The listing builds one solid part. Answer for the finished solid, in the listing's coordinates (mm). A direction names the side the tool comes from. Coordinates: 2 decimals unless noted, no trailing zeros. Loops run counter-clockwise (first coordinate to the right, second up) from the corner with the lowest first, then second, coordinate; pieces in that order, holes last. Notation, with made-up numbers: (-9.5, 0.5) - (36.5, 0.5) arc R26 ccw to (36.5, 28.5) - close; hole circle Ø11 at (-33.5, 42). An arc over 180 degrees is marked (long way). Return JSON: item names as keys, results as strings. Group by question number.
1. Section B-B (z = 402) is taken. Write down the section's boundary in (x, y), and give its area (3 significant figures).
2. Which of the six approach directions +Z, -Z, +X, -X, +Y, -Y give full straight-line access (tool end or side, diameter ignored) to faces 4 (the face through (31.75, 16, 363)), 5 (the face through (6.35, 16, 363))?
3. Find the intervals of material crossed by line 1 along X through (y, z) = (20.5, 138.5); line 2 along Z through (x, y) = (15.5, 26.5), in increasing order.
4. The mould has two halves that part along Y. Classify faces 1 (the face through (0, 16, 363)), 2 (the face through (16, 25.4, 363)), 3 (the face through (16, 31.75, 363)): pulls with the +Y half, pulls with the -Y half, needs draft (parallel to the pull), parting line crosses it, or undercut.
5. Each of these flat-tipped pins is pushed along its axis until it touches: P1, Ø7.5, axis at x = 15.875, z = 25.4, coming from the -Y side; P2, Ø8, axis at x = 8.5, y = 8.5, coming from the -Z side. Where does it stop, or does it pass through?
```python
from build123d import *

# Parameters (mm, degrees)
F0_W     = 31.75
F0_H     = 31.75
F0_W_2   = 19.05
F0_H_2   = 19.05
F1_DEPTH = 736.6
F2_R     = 4.7625
F3_DEPTH = 31.751
F5_DEPTH = 31.751


with BuildPart() as f1:
    # F0 (on Top) → F1 (new body)
    with BuildSketch(Plane.XY):
        with Locations((15.875, 15.875)):
            Rectangle(F0_W, F0_H)
        with Locations((15.875, 15.875)):
            Rectangle(F0_W_2, F0_H_2, mode=Mode.SUBTRACT)
    extrude(amount=F1_DEPTH)

    # F2 (on face) → F3 (cut, through all)
    with BuildSketch(Plane.XZ):
        with Locations((15.875, 25.4)):
            Circle(F2_R)
    extrude(amount=-F3_DEPTH, mode=Mode.SUBTRACT)

    # F4 (on face) → F5 (cut, through all)
    with BuildSketch(Plane.XZ):
        with BuildLine():
            ThreePointArc((27.532244, 727.619744), (27.16972, 729.442274), (26.13734, 730.98734))
            ThreePointArc((26.13734, 730.98734), (18.369768, 725.797214), (27.532244, 727.619744))
        make_face()
    extrude(amount=-F5_DEPTH, mode=Mode.SUBTRACT)


solid = f1.part
```
The answers:
{
 "1": {"outline": "(0, 0) - (31.75, 0) - (31.75, 31.75) - (0, 31.75) - close; hole (6.35, 6.35) - (25.4, 6.35) - (25.4, 25.4) - (6.35, 25.4) - close", "area": "645 mm2"},
 "2": {"face 4": "+Z, -Z, +X, +Y, -Y", "face 5": "+Z, -Z"},
 "3": {"line 1": "x = 0 to 6.35, 25.4 to 31.75", "line 2": "z = 0 to 20.65, 30.15 to 736.6"},
 "4": {"face 1": "needs draft", "face 2": "undercut", "face 3": "pulls with the +Y half"},
 "5": {"P1": "passes through", "P2": "stops at z = 0"}
}
